Model file for the job. Use its own axes, mm. A direction names the side the tool comes from. Round coordinates to 2 decimals unless told otherwise and drop trailing zeros. Order: outer loops, then holes, each group sorted by start corner. A loop starts at its lowest first (then second) coordinate and runs counter-clockwise, first axis right, second up. Notation, with made-up numbers: (-1, -37.5) - (15, -37.5) arc R22 ccw to (15, -19.5) - close; hole circle Ø9 at (6, 16.25). An arc over 180 degrees is marked (long way). Use one line per item in the form item = value.
from build123d import *

# Parameters (mm, degrees)
SKETCH2_W           = 10
SKETCH2_H           = 15
BOSS_EXTRUDE1_DEPTH = 81.5
SKETCH2_3_W         = 10
SKETCH2_3_H         = 15
BOSS_EXTRUDE2_DEPTH = 21
FILLET1_R           = 5


with BuildPart() as part:
    # Sketch2 → Boss-Extrude1 (new body)
    with BuildSketch(Plane(origin=(0, 0, 0), x_dir=(1, 0, 0), z_dir=(0, 1, 0))):
        Polygon((-11.5, 11.5), (-11.5, -11.5), (-5, -11.5), (-5, 3.5), (5, 3.5), (5, -11.5), (11.5, -11.5), (11.5, 11.5), align=None)
        with Locations((0, -4)):
            Rectangle(SKETCH2_W, SKETCH2_H)
    extrude(amount=BOSS_EXTRUDE1_DEPTH)

    # Sketch2_3 → Boss-Extrude2 (add)
    with BuildSketch(Plane(origin=(0, 0, 0), x_dir=(1, 0, 0), z_dir=(0, 1, 0))):
        with Locations((0, -4)):
            Rectangle(SKETCH2_3_W, SKETCH2_3_H)
    boss_extrude2 = extrude(amount=-BOSS_EXTRUDE2_DEPTH)

    # Fillet1
    fillet1_edges = [part.edges().sort_by_distance(p)[0] for p in [
        (-11.5, 40.75, -11.5),
        (11.5, 40.75, -11.5),
        (11.5, 40.75, 11.5),
        (-11.5, 40.75, 11.5),
    ]]
    fillet(fillet1_edges, radius=FILLET1_R)

    # Mirror1: Boss-Extrude2 across plane
    add(boss_extrude2.mirror(Plane.ZX.offset(40.486123935)))


solid = part.part
(1) Slice it at C-C on y = 37. Give the cut face in (x, z), then the cut area to 3 significant figures.
Report:
outline = (-11.5, -6.5) arc R5 ccw to (-6.5, -11.5) - (6.5, -11.5) arc R5 ccw to (11.5, -6.5) - (11.5, 6.5) arc R5 ccw to (6.5, 11.5) - (-6.5, 11.5) arc R5 ccw to (-11.5, 6.5) - close
area = 508 mm2
(2) Pin check, flat tips, straight feed: pin 1 (7.5 mm diameter, centred on y = 89, z = 5, fed in from -X); pin 2 (1.5 mm diameter, centred on x = -6.5, z = 7, fed in from +Y); pin 3 (5 mm diameter, centred on y = 86.5, z = -7, fed in from -X); pin 4 (7.5 mm diameter, centred on y = -12.5, z = 7, fed in from +X). Stop position of each tip, or through.
Report:
pin_1 = -5
pin_2 = 81.5
pin_3 = through
pin_4 = 5
(3) Tool access for faces 1 (the face through (0, 92, -3.5)), 2 (the face through (-5, -10, 4)), 3 (the face through (-5, 92, 4)), 4 (the face through (0, -10, -3.5)): list every direction of +Z, -Z, +X, -X, +Y, -Y with a clear straight run to the whole face (end or side of a thin tool).
Report:
face_1 = -Z, +X, -X, +Y
face_2 = +Z, -Z, -X, -Y
face_3 = +Z, -Z, -X, +Y
face_4 = -Z, +X, -X, -Y
(4) Slice it at D-D on z = 9. Give the cut face in (x, y).
Report:
outline = (-10.83, 0) - (-5, 0) - (-5, -21) - (5, -21) - (5, 0) - (10.83, 0) - (10.83, 81.5) - (5, 81.5) - (5, 101.97) - (-5, 101.97) - (-5, 81.5) - (-10.83, 81.5) - close
(5) Slice it at B-B on z = 4. Give the cut face in (x, y).
Report:
outline = (-11.5, 0) - (-5, 0) - (-5, -21) - (5, -21) - (5, 0) - (11.5, 0) - (11.5, 81.5) - (5, 81.5) - (5, 101.97) - (-5, 101.97) - (-5, 81.5) - (-11.5, 81.5) - close
(6) Probe probe 1 along Y at (x, z) = (9.5, -3); probe 2 along X at (y, z) = (85, 8.5); probe 3 along Z at (x, y) = (1.5, 94.5). List the from-to ranges inside material, lowest first. Write a range as [from, to].
Report:
probe_1 = [0, 81.5]
probe_2 = [-5, 5]
probe_3 = [-3.5, 11.5]
(7) Slice it at A-A on x = 1.25. Give the cut face in (y, z).
Report:
outline = (-21, -3.5) - (0, -3.5) - (0, -11.5) - (81.5, -11.5) - (81.5, -3.5) - (101.97, -3.5) - (101.97, 11.5) - (-21, 11.5) - close
